Model file for the job. Use its own axes, mm. A direction names the side the tool comes from. Round coordinates to 2 decimals unless told otherwise and drop trailing zeros. Order: outer loops, then holes, each group sorted by start corner. A loop starts at its lowest first (then second) coordinate and runs counter-clockwise, first axis right, second up. Notation, with made-up numbers: (56, 27.25) -> (104, 27.25) arc R19 ccw to (104, 58.25) -> close; hole circle Ø7 at (60, 89.5). An arc over 180 degrees is marked (long way). Use CSV: the item, a comma, the result in double quotes.
```python
from build123d import *

# Parameters (mm, degrees)
SKETCH1_W        = 270
SKETCH1_H        = 180
EXTRUDE1_DEPTH   = 180
FILLET1_R        = 10
SHELL1_START     = -125
SHELL1_OUTLINE_W = 170
SHELL1_OUTLINE_H = 160
SHELL1_DEPTH     = 250
SKETCH2_W        = 65
SKETCH2_H        = 65
EXTRUDE2_DEPTH   = 20
FILLET2_R        = 3


# Read off the part's stored shape, not the designer's step: Shell1
with BuildPart() as part:
    # Sketch1 → Extrude1 (new body)
    with BuildSketch(Plane(origin=(0, 0, 0), x_dir=(1, 0, 0), z_dir=(0, 1, 0))):
        Rectangle(SKETCH1_W, SKETCH1_H)
    extrude(amount=EXTRUDE1_DEPTH)

    # Fillet1
    fillet1_edges = [part.edges().sort_by_distance(p)[0] for p in [
        (0, 0, 90),
        (-135, 0, 0),
        (0, 0, -90),
        (135, 0, 0),
        (135, 90, 90),
        (-135, 90, 90),
        (-135, 90, -90),
        (135, 90, -90),
    ]]
    fillet(fillet1_edges, radius=FILLET1_R)

    # Shell1 outline → Shell1 (cut)
    with BuildSketch(Plane.YZ.offset(SHELL1_START)):
        with Locations((95, 0)):
            Rectangle(SHELL1_OUTLINE_W, SHELL1_OUTLINE_H)
    extrude(amount=SHELL1_DEPTH, mode=Mode.SUBTRACT)

    # Sketch2 → Extrude2 (cut)
    with BuildSketch(Plane.XY.offset(90)):
        with Locations((-62.5, 127.5)):
            Rectangle(SKETCH2_W, SKETCH2_H)
    extrude(amount=-EXTRUDE2_DEPTH, mode=Mode.SUBTRACT)

    # Fillet2
    fillet2_edges = [part.edges().sort_by_distance(p)[0] for p in [
        (-62.5, 95, 90),
        (-30, 127.5, 90),
        (-62.5, 160, 90),
    ]]
    fillet(fillet2_edges, radius=FILLET2_R)


solid = part.part
```
Q1. Which spindle directions (+Z, -Z, +X, -X, +Y, -Y) get a long thin tool onto all of the face, cutting with end or side? Do faces 1 (the flat face through (-125, 94, 1)), 2 (the flat face through (-30, 127, 84)), 3 (the flat face through (-2, 94, -90)). Say none if no direction does.
From the geometry:
face 1,"+Y"
face 2,"+Z"
face 3,"-Z, +X, -X, +Y, -Y"
Q2. Pin check, flat tips, straight feed: pin 1 (2 mm diameter, centred on x = -89, z = 42, fed in from +Y); pin 2 (11 mm diameter, centred on y = 135, z = 86.5, fed in from +X); pin 3 (2 mm diameter, centred on y = 133, z = 83.5, fed in from -X). Stop position of each tip, or through.
From the geometry:
pin 1,"stops at y = 10"
pin 2,"stops at x = 134.95"
pin 3,"stops at x = -134.68"
Q3. Cut at A-A (x = -52.5). Give the cut face in (y, z).
From the geometry:
outline,"(0, -80) arc R10 ccw to (10, -90) -> (180, -90) -> (180, -80) -> (10, -80) -> (10, 80) -> (95, 80) -> (95, 87) arc R3 ccw to (92, 90) -> (10, 90) arc R10 ccw to (0, 80) -> close; (160, 80) -> (180, 80) -> (180, 90) -> (163, 90) arc R3 ccw to (160, 87) -> close"
Q4. Cut at B-B (y = 56). Give the cut face in (x, z).
From the geometry:
outline,"(-135, -80) arc R10 ccw to (-125, -90) -> (125, -90) arc R10 ccw to (135, -80) -> (135, 80) arc R10 ccw to (125, 90) -> (-125, 90) arc R10 ccw to (-135, 80) -> close; hole (-125, -80) -> (125, -80) -> (125, 80) -> (-125, 80) -> close"
Q5. Cut at C-C (z = 24). Give the cut face in (x, y), plus the area to 3 significant figures.
From the geometry:
outline,"(-135, 10) arc R10 ccw to (-125, 0) -> (125, 0) arc R10 ccw to (135, 10) -> (135, 180) -> (125, 180) -> (125, 10) -> (-125, 10) -> (-125, 180) -> (-135, 180) -> close"
area,"6,060 mm²"
Q6. Mould opens along Z. For faces 4 (the flat face through (-95, 127, 85)), 5 (the cylindrical face through (1.75, 3.01, 87.15)), 6 (the flat face through (-2, 94, -80)) say: +Z half, -Z half, draft (parallel to the pull), parting line (faces both ways), or undercut.
From the geometry:
face 4,"draft"
face 5,"+Z half"
face 6,"undercut"
Q7. Probe line 1 along Z through (x, y) = (85, 94); line 2 along X through (y, z) = (135.5, -8.5); line 3 along Y through (x, z) = (93, 22). List the from-to ranges inside material, lowest first.
From the geometry:
line 1,"z = -90 to -80, 80 to 90"
line 2,"x = -135 to -125, 125 to 135"
line 3,"y = 0 to 10"
Q8. Cut at D-D (x = 74). Give the cut face in (y, z), plus the area to 3 significant figures.
From the geometry:
outline,"(0, -80) arc R10 ccw to (10, -90) -> (180, -90) -> (180, -80) -> (10, -80) -> (10, 80) -> (180, 80) -> (180, 90) -> (10, 90) arc R10 ccw to (0, 80) -> close"
area,"5,160 mm²"
